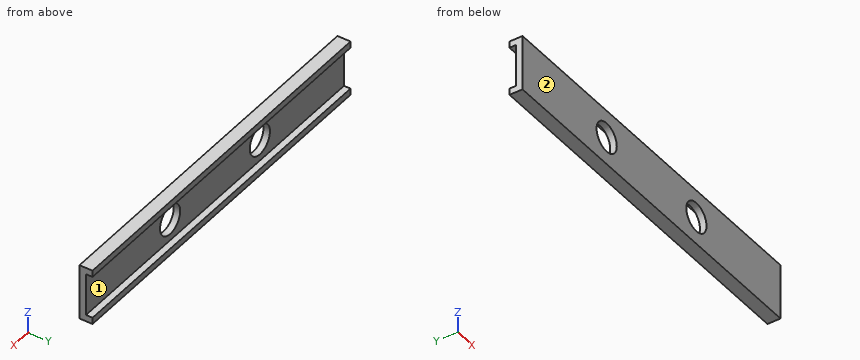
from build123d import *

# Parameters (mm, degrees)
SKETCH5_R               = 9
F_2_STK_18_HULLER_DEPTH = 13.167105011
SKETCH3_W               = 62.936012514
SKETCH3_H               = 32.167105011
DUMMY_CUT_AWAY1_DEPTH   = 35
SKETCH6_W               = 62.936012514
SKETCH6_H               = 32.167105011
DUMMY_CUT_AWAY2_DEPTH   = 35
DUMMY_RET1_DEPTH        = 65


with BuildPart() as part:
    # Sweep1: sweep along a path in Sketch1
    with BuildLine(Plane.XY) as sweep1_path:
        Line((-225.364862075, -4.470649394), (-218.416595736, 1.359638329))
        ThreePointArc((-218.416595736, 1.359638329), (-214.807386139, 3.443416461), (-210.703144419, 4.167105011))
        Line((-210.703144419, 4.167105011), (-188.097668128, 4.167105011))
        ThreePointArc((-188.097668128, 4.167105011), (-186.013889996, 3.984798048), (-183.993426408, 3.443416461))
        Line((-183.993426408, 3.443416461), (-177.3495012, 1.025225447))
        ThreePointArc((-177.3495012, 1.025225447), (-174.487177784, 0.258268199), (-171.535158764, 0))
        Line((-171.535158764, 0), (-58.464841236, 0))
        ThreePointArc((-58.464841236, 0), (-55.512822216, 0.258268199), (-52.6504988, 1.025225447))
        Line((-52.6504988, 1.025225447), (-46.006573592, 3.443416461))
        ThreePointArc((-46.006573592, 3.443416461), (-43.986110004, 3.984798048), (-41.902331872, 4.167105011))
        Line((-41.902331872, 4.167105011), (-19.296855581, 4.167105011))
        ThreePointArc((-19.296855581, 4.167105011), (-15.192613861, 3.443416461), (-11.583404264, 1.359638329))
        Line((-11.583404264, 1.359638329), (-4.635137925, -4.470649394))
    # Sketch2 → Sweep1 (sweep)
    with BuildSketch(Plane(origin=(-4.635137925, -4.470649394, 0), x_dir=(0, 0, -1), z_dir=(0.766044443, -0.64278761, 0))):
        Polygon((0, 0), (0.5, 0), (0.5, 4), (4.5, 4), (4.5, -4), (-29.5, -4), (-29.5, 4), (-25.5, 4), (-25.5, 0), align=None)
    sweep(path=sweep1_path.line)

    # Sketch5 → 2 stk ø18 huller (cut, through all)
    with BuildSketch(Plane.XZ.offset(4)):
        with Locations((-75, 12.5)):
            Circle(SKETCH5_R)
        with Locations((-155, 12.5)):
            Circle(SKETCH5_R)
    extrude(amount=-F_2_STK_18_HULLER_DEPTH, mode=Mode.SUBTRACT)

    # Sketch3 → Dummy cut away1 (cut, through all)
    with BuildSketch(Plane.XY.offset(29.5)):
        with Locations((-33.531993743, 2.083552506)):
            Rectangle(SKETCH3_W, SKETCH3_H)
    extrude(amount=-DUMMY_CUT_AWAY1_DEPTH, mode=Mode.SUBTRACT)

    # Sketch6 → Dummy cut away2 (cut, through all)
    with BuildSketch(Plane.XY.offset(29.5)):
        with Locations((-196.468006257, 2.083552506)):
            Rectangle(SKETCH6_W, SKETCH6_H)
    extrude(amount=-DUMMY_CUT_AWAY2_DEPTH, mode=Mode.SUBTRACT)

    # Sketch4 → Dummy ret1 (add)
    with BuildSketch(Plane.ZY.offset(165)):
        Polygon((29.5, -4), (29.5, 4), (25.5, 4), (25.5, 0), (-0.5, 0), (-0.5, 4), (-4.5, 4), (-4.5, -4), align=None)
    dummy_ret1 = extrude(amount=DUMMY_RET1_DEPTH)

    # Mirror1: Dummy ret1 across plane
    add(dummy_ret1.mirror(Plane(origin=(-115, 4, 29.5), x_dir=(0, 0, 1), z_dir=(-1, 0, 0))))


solid = part.part
Can you work these out from the model? Positions are in its coordinate system, mm. Face numbers are marked on the shaded views. Give positions to 0.01 mm unless a question says otherwise; leave off trailing zeros. Order: outer loops, then holes, each group sorted by start corner. A loop starts at its lowest first (then second) coordinate and runs counter-clockwise, first axis right, second up. Notation, with made-up numbers: M 58,-29 L 79,-29 A13 cw 79,-20 Z; hole C 82,28.5 d4. An arc over 180 degrees is marked long. Use one line per item in the form item = value.
Item 1: If we section it at D-D, the plane x = -24.5: Write out the boundary of the cut face in (y, z), and give its area (3 significant figures).
Values follow:
outline = M -4,-4.5 L 4,-4.5 L 4,-0.5 L 0,-0.5 L 0,25.5 L 4,25.5 L 4,29.5 L -4,29.5 Z
area = 168 mm^2
Item 2: If we section it at B-B, the plane z = 5.5: Write out the boundary of the cut face in (x, y), and give its area (3 significant figures).
Values follow:
outline = M -230,-4 L -160.66,-4 L -160.66,0 L -230,0 Z; M -149.34,-4 L -80.66,-4 L -80.66,0 L -149.34,0 Z; M -69.34,-4 L 0,-4 L 0,0 L -69.34,0 Z
area = 829 mm^2
Item 3: Will these pins go through, and if not, where does the flat tip stop? pin 1 Ø11 at (x, z) = (-75, 12.5) entering from -Y; pin 2 Ø1 at (x, z) = (-134.5, 0.5) entering from +Y; pin 3 Ø8 at (x, z) = (-158.5, 7) entering from -Y.
Values follow:
pin_1 = through
pin_2 = 0
pin_3 = -4
Item 4: If we section it at A-A, the plane x = -75: Write out the boundary of the cut face in (y, z), and give its area (3 significant figures).
Values follow:
outline = M -4,-4.5 L 4,-4.5 L 4,-0.5 L 0,-0.5 L 0,3.5 L -4,3.5 Z; M -4,21.5 L 0,21.5 L 0,25.5 L 4,25.5 L 4,29.5 L -4,29.5 Z
area = 96.0 mm^2
Item 5: If I drill on line 1 along Z through (x, y) = (-150, 1); line 2 along Z through (x, y) = (-75, -0.9); line 3 along Y through (x, z) = (-128, 20.5), over which ranges is the centre line in solid material (lowest first)? Write a range as [from, to].
Values follow:
line_1 = [-4.5, -0.5], [25.5, 29.5]
line_2 = [-4.5, 3.5], [21.5, 29.5]
line_3 = [-4, 0]
Item 6: Thinking about a two-plate mould opening in Z: for the marked faces 1 and 2, which applies, pulls with the +Z half, pulls with the -Z half, needs draft (parallel to the pull), parting line crosses it, or undercut?
Values follow:
face_1 = undercut
face_2 = needs draft
Item 7: If we section it at C-C, the plane y = -1.5: Write out the boundary of the cut face in (x, z).
Values follow:
outline = M -230,-4.5 L 0,-4.5 L 0,29.5 L -230,29.5 Z; hole C -155,12.5 d18; hole C -75,12.5 d18
